Print and shaded views of the part. All mm, measured from the part's lowest x, y and z. A direction names the side the tool comes from. Round coordinates to 2 decimals unless told otherwise and drop trailing zeros. Write each loop counter-clockwise with the first axis right and the second up, starting at its lowest first coordinate (ties: lowest second). Pieces come first, ordered by that corner, then holes. Notation, with made-up numbers: M -33.5,32 L 25.5,32 A22 cw 25.5,40 Z; hole C -15,27 d1. An arc over 180 degrees is marked long. Write item = value, one per line. Start each with the question number.
Q1. Band-saw the part on B-B on z = 24.5. Write the cut outline in (x, y) (3 decimals), plus the area to 3 significant figures.
Q2. Drop a flat-ended pin along its axis: P1, Ø2, axis at x = 226.5, y = 112, coming from the +Z side. Give the stop position or say it passes through.
Q3. Band-saw the part on C-C on y = 97.5. Write the cut outline in (x, z) (3 decimals).
Q4. Probe L1, parallel to X at y = 105.5, z = 18 (3 decimals); L2, parallel to Y at x = 285, z = 60.5 (3 decimals); L3, parallel to Y at x = 198, z = 49.5 (3 decimals). List the from-to ranges inside material, lowest first.
Q5. Tool access for the marked faces 4, 5 and 6: list every direction of +Z, -Z, +X, -X, +Y, -Y with a clear straight run to the whole face (end or side of a thin tool).
Q6. Pull direction Y, two halves, no side cores. Call the marked faces 1, 2 and 3: released by +Y, released by -Y, zero draft, split by the parting line, or undercut.
Q7. Band-saw the part on D-D on x = 54. Write the cut outline in (y, z) (3 decimals), plus the area to 3 significant figures.
Q8. Band-saw the part on A-A on x = 196.5. Write the cut outline in (y, z) (3 decimals), plus the area to 3 significant figures.
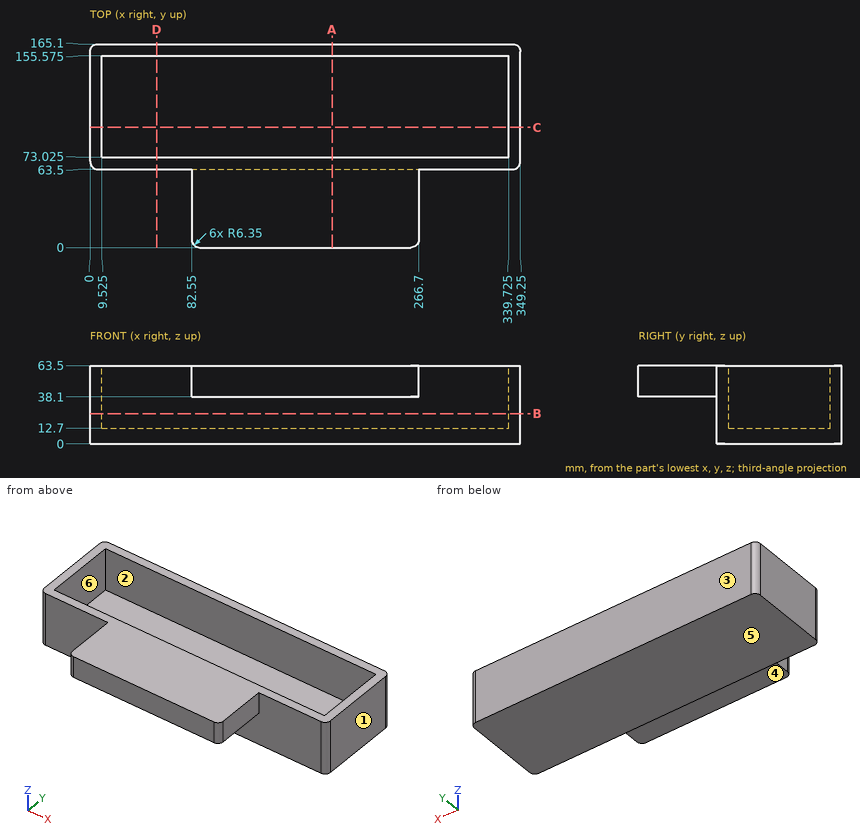
Conclusion:
q1.outline = M 0,69.85 A6.35 ccw 6.35,63.5 L 342.9,63.5 A6.35 ccw 349.25,69.85 L 349.25,158.75 A6.35 ccw 342.9,165.1 L 6.35,165.1 A6.35 ccw 0,158.75 Z; hole M 9.525,73.025 L 339.725,73.025 L 339.725,155.575 L 9.525,155.575 Z
q1.area = 8,190 mm^2
q2.P1 = 12.7
q3.outline = M 0,0 L 349.25,0 L 349.25,63.5 L 339.725,63.5 L 339.725,12.7 L 9.525,12.7 L 9.525,63.5 L 0,63.5 Z
q4.L1 = 0 to 9.525, 339.725 to 349.25
q4.L2 = 63.5 to 73.025, 155.575 to 165.1
q4.L3 = 0 to 73.025, 155.575 to 165.1
q5.face_4 = -Z, +X, -X, -Y
q5.face_5 = -Z, +X, -X, +Y, -Y
q5.face_6 = +Z
q6.face_1 = zero draft
q6.face_2 = undercut
q6.face_3 = released by +Y
q7.outline = M 63.5,0 L 165.1,0 L 165.1,63.5 L 155.575,63.5 L 155.575,12.7 L 73.025,12.7 L 73.025,63.5 L 63.5,63.5 Z
q7.area = 2,260 mm^2
q8.outline = M 0,38.1 L 63.5,38.1 L 63.5,0 L 165.1,0 L 165.1,63.5 L 155.575,63.5 L 155.575,12.7 L 73.025,12.7 L 73.025,63.5 L 0,63.5 Z
q8.area = 3,870 mm^2
